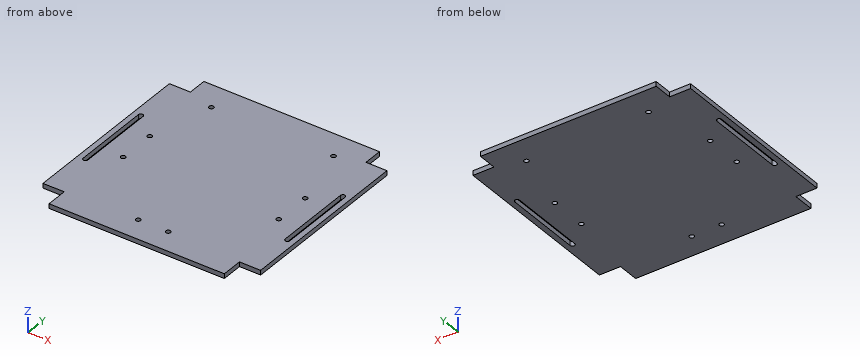
from build123d import *

# Parameters (mm, degrees)
F0_W      = 70
F0_H      = 140
F1_DEPTH  = 3
F3_D      = 3
F9_D      = 3
F11_D     = 3
F12_W     = 13.50167
F12_H     = 12.155368
F13_DEPTH = 3
F14_W     = 13.607755
F14_H     = 13.643959
F15_DEPTH = 4.788373
F16_DEPTH = 36.920227


with BuildPart() as f1:
    # F0 (on Top) → F1 (new body)
    with BuildSketch(Plane.XY):
        with Locations((35, 70)):
            Rectangle(F0_W, F0_H)
    extrude(amount=F1_DEPTH)

    # F3 (through all)
    with Locations(Plane.XY.offset(3)):
        with Locations((50, 58), (50, 82)):
            Hole(F3_D / 2)

    # F9 (through all)
    with Locations(Plane.XY.offset(3)):
        with Locations((39.273195, 122.702248)):
            Hole(F9_D / 2)

    # F11 (through all)
    with Locations(Plane.XY.offset(3)):
        with Locations((9.616546, 14.959589)):
            Hole(F11_D / 2)

    # F12 (on face) → F13 (cut)
    with BuildSketch(Plane.XY.offset(3)):
        with Locations((63.249165, 133.922316)):
            Rectangle(F12_W, F12_H)
    extrude(amount=-F13_DEPTH, mode=Mode.SUBTRACT)

    # F14 (on face) → F15 (cut)
    with BuildSketch(Plane.XY.offset(3)):
        with Locations((63.196123, 6.821979)):
            Rectangle(F14_W, F14_H)
    extrude(amount=-F15_DEPTH, mode=Mode.SUBTRACT)

    # F7 (on face) → F16 (cut)
    with BuildSketch(Plane.XY.offset(3)):
        with BuildLine():
            ThreePointArc((63.5, 45), (65, 43.5), (66.5, 45))
            Line((66.5, 45), (66.5, 95))
            ThreePointArc((66.5, 95), (65, 96.5), (63.5, 95))
            Line((63.5, 95), (63.5, 45))
        make_face()
    extrude(amount=-F16_DEPTH, mode=Mode.SUBTRACT)

    # F17: F1 across plane


with BuildPart() as f1_1:
    add(f1.part)
    add(f1.part.mirror(Plane.YZ))


solid = f1_1.part
Geometry: final body of the model. Coordinates: model frame, mm. Round coordinates to 2 decimals unless told otherwise and drop trailing zeros. Order: outer loops, then holes, each group sorted by start corner. A loop starts at its lowest first (then second) coordinate and runs counter-clockwise, first axis right, second up.
Q1. Section B-B, the plane z = 2.05. Give the number of separate pieces and of enclosed holes in the cut face, and give its area (3 significant figures).
Result sheet:
separate pieces: 1
enclosed holes: 10
area: 18,500 mm2
Q2. Material intervals for probe 1 along X at (y, z) = (55, 0.65); probe 2 along X at (y, z) = (82, 0.9); probe 3 along Y at (x, z) = (50, 1.45), sorted ascending.
Result sheet:
probe 1: x = -70 to -66.5, -63.5 to 63.5, 66.5 to 70
probe 2: x = -70 to -66.5, -63.5 to -51.5, -48.5 to 48.5, 51.5 to 63.5, 66.5 to 70
probe 3: y = 0 to 56.5, 59.5 to 80.5, 83.5 to 140
Q3. Section A-A, the plane y = 61.5. Output: boundary loops of the cut face in (x, z).
Result sheet:
outline: (-70, 0) - (-66.5, 0) - (-66.5, 3) - (-70, 3) - close; (-63.5, 0) - (63.5, 0) - (63.5, 3) - (-63.5, 3) - close; (66.5, 0) - (70, 0) - (70, 3) - (66.5, 3) - close
Q4. Pin query (flat end, axial travel): pin 1 (1.5 mm diameter, centred on y = 131, z = 1.5, fed in from +X); pin 2 (2.5 mm diameter, centred on x = -50, y = 58, fed in from +Z); pin 3 (0.9 mm diameter, centred on x = -64, z = 1, fed in from +Y). Return the tip coordinate at first contact, or that it passes through.
Result sheet:
pin 1: stops at x = 56.5
pin 2: passes through
pin 3: stops at y = 127.84
